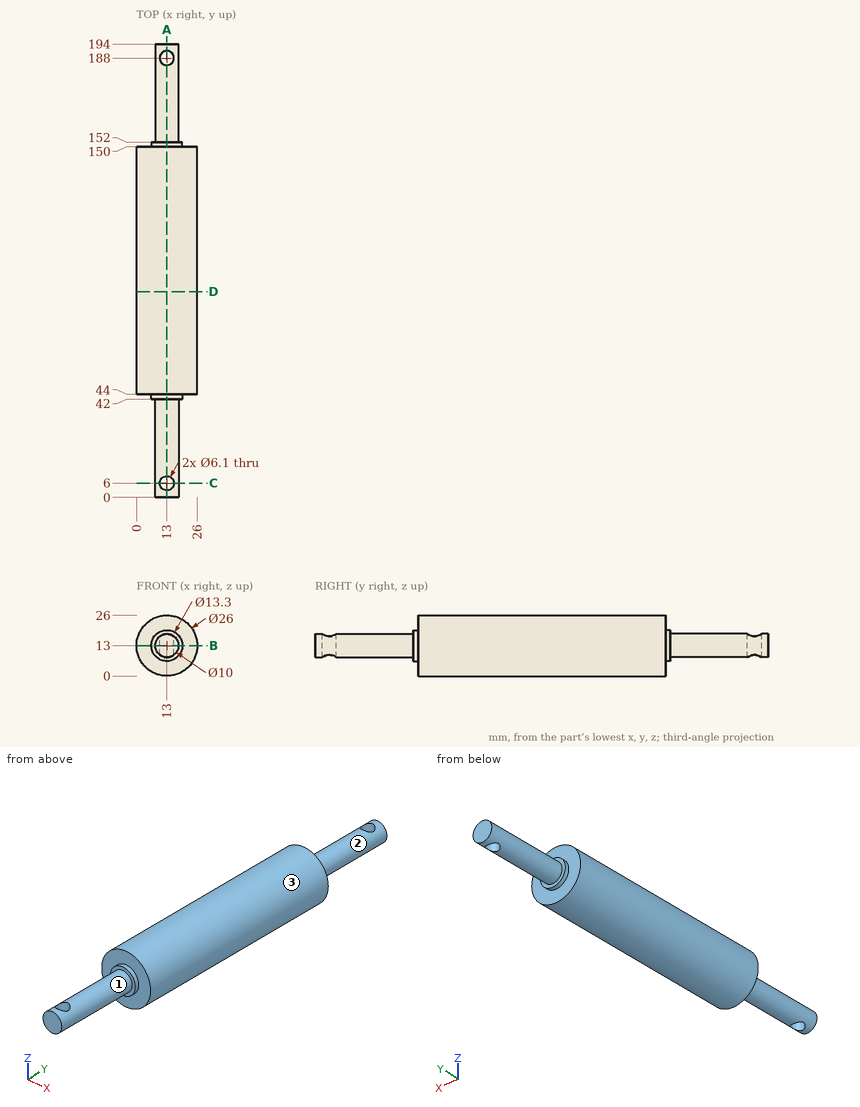
Input: dimensioned drawing with shaded views. Units: mm. Origin: part minimum x, y, z. A direction names the side the tool comes from. Round coordinates to 2 decimals unless told otherwise and drop trailing zeros. Loops run counter-clockwise (first coordinate to the right, second up) from the corner with the lowest first, then second, coordinate; pieces in that order, holes last. Notation, with made-up numbers: M 83.25,-39.75 L 121.25,-39.75 A12 cw 121.25,-25.75 Z; hole C -28.5,-10 d2. An arc over 180 degrees is marked long. Answer in a Markdown table with one row per item. Add a question column.
1. Section D-D (y = 88). Output: boundary loops of the cut face in (x, z), and give its area (3 significant figures).
2. Ray query, probe 1 along Y at (x, z) = (13, 15.5); probe 2 along Y at (x, z) = (14.75, 15.5); probe 3 along Y at (x, z) = (17.5, 22.25). Return the intervals inside material, ascending.
3. Contact query for flat-ended pins moving along their axis: pin 1 (2 mm diameter, centred on x = 17.5, y = 135, fed in from -Z); pin 2 (1 mm diameter, centred on y = 67.5, z = 16, fed in from -X); pin 3 (6 mm diameter, centred on y = 68, z = 3.5, fed in from -X); pin 4 (5 mm diameter, centred on x = 13, y = 188, fed in from +Z). Output: stop coordinate, or through.
4. Set-up query: the marked faces 1, 2 and 3. Return all of +Z, -Z, +X, -X, +Y, -Y with unobstructed straight access to the full face (end or side cutting, diameter ignored); none if empty.
5. Section C-C (y = 6). Output: boundary loops of the cut face in (x, z).
6. Section A-A (x = 13). Output: boundary loops of the cut face in (y, z).
7. Section B-B (z = 13). Output: boundary loops of the cut face in (x, y), and give its area (3 significant figures).
Values follow:
| question | item | result |
|---|---|---|
| 1 | outline | C 13,13 d26 |
| 1 | area | 531 mm^2 |
| 2 | probe 1 | 0 to 2.95, 9.05 to 184.95, 191.05 to 194 |
| 2 | probe 2 | 0 to 3.5, 8.5 to 185.5, 190.5 to 194 |
| 2 | probe 3 | 44 to 150 |
| 3 | pin 1 | z = 0.48 |
| 3 | pin 2 | x = 0.24 |
| 3 | pin 3 | x = 1.74 |
| 3 | pin 4 | through |
| 4 | face 1 | -Y |
| 4 | face 2 | +Y |
| 4 | face 3 | +Y, -Y |
| 5 | outline | M 9.95,9.04 L 9.95,16.96 A5 ccw Z; M 16.05,9.04 A5 ccw 16.05,16.96 Z |
| 6 | outline | M 0,8 L 2.95,8 L 2.95,18 L 0,18 Z; M 9.05,8 L 42,8 L 42,6.35 L 44,6.35 L 44,0 L 150,0 L 150,6.35 L 152,6.35 L 152,8 L 184.95,8 L 184.95,18 L 152,18 L 152,19.65 L 150,19.65 L 150,26 L 44,26 L 44,19.65 L 42,19.65 L 42,18 L 9.05,18 Z; M 191.05,8 L 194,8 L 194,18 L 191.05,18 Z |
| 7 | outline | M 0,44 L 6.35,44 L 6.35,42 L 8,42 L 8,0 L 18,0 L 18,42 L 19.65,42 L 19.65,44 L 26,44 L 26,150 L 19.65,150 L 19.65,152 L 18,152 L 18,194 L 8,194 L 8,152 L 6.35,152 L 6.35,150 L 0,150 Z; hole C 13,6 d6.1; hole C 13,188 d6.1 |
| 7 | area | 3,590 mm^2 |
